Geometry check sheet. Reference: the model listing, model coordinates, mm. A direction names the side the tool comes from. Coordinates: 2 decimals unless noted, no trailing zeros. Write each loop counter-clockwise with the first axis right and the second up, starting at its lowest first coordinate (ties: lowest second). Pieces come first, ordered by that corner, then holes. Notation, with made-up numbers: M 71,66 L 80,66 A32 ccw 80,100 Z; hole C 44.5,42 d3. An arc over 180 degrees is marked long. Write item = value, one per line. Start each with the question number.
```python
from build123d import *

# Parameters (mm, degrees)
SZKIC1_R                    = 40
DODANIE_WYCI_GNI_CIE1_DEPTH = 300
DODANIE_WYCI_GNI_CIE2_DEPTH = 40
SZKIC3_R                    = 30
WYTNIJ_WYCI_GNI_CIE1_DEPTH  = 81


with BuildPart() as part:
    # Szkic1 → Dodanie-wyciągnięcie1 (new body)
    with BuildSketch(Plane.XY):
        Circle(SZKIC1_R)
    extrude(amount=DODANIE_WYCI_GNI_CIE1_DEPTH)

    # Szkic2 → Dodanie-wyciągnięcie2 (add, symmetric)
    with BuildSketch(Plane(origin=(0, 0, 0), x_dir=(0, 0, -1), z_dir=(1, 0, 0))):
        with BuildLine():
            Line((-340, -40), (-300, -40))
            Line((-300, -40), (-300, 40))
            Line((-300, 40), (-340, 40))
            ThreePointArc((-340, 40), (-380, 0), (-340, -40))
        make_face()
    extrude(amount=DODANIE_WYCI_GNI_CIE2_DEPTH, both=True)

    # Szkic3 → Wytnij-wyciągnięcie1 (cut, through all)
    with BuildSketch(Plane(origin=(40, 0, 0), x_dir=(0, 0, -1), z_dir=(1, 0, 0))):
        with Locations((-340, 0)):
            Circle(SZKIC3_R)
    extrude(amount=-WYTNIJ_WYCI_GNI_CIE1_DEPTH, mode=Mode.SUBTRACT)


solid = part.part
```
Q1. Set-up check for faces 1 (the face through (-32, 32, 300)), 2 (the face through (-8.67, -39.05, 147.9)), 3 (the face through (-30, -32, 300)), 4 (the face through (32, 30, 300)): record each of +Z, -Z, +X, -X, +Y, -Y from which the full face is reachable in a straight line by a thin tool's end or side.
Q2. Cross-section at A-A on y = -16.5. Enter the section's corners in (x, z), and give its area (3 significant figures).
Q3. Scan lines: L1, parallel to Y at x = 3, z = 340; L2, parallel to Y at x = 36, z = 358; L3, parallel to Z at x = -32.5, y = 7.5. Record each from-to range of solid material in increasing order.
Q4. Cross-section at C-C on z = 138.5. Enter the section's corners in (x, y), and give its area (3 significant figures).
Q5. Gauge pin test, flat ends, axial feed: pin 1 (3 mm diameter, centred on y = -26, z = 126, fed in from +X); pin 2 (1.5 mm diameter, centred on y = 26.5, z = 102.5, fed in from -X); pin 3 (3 mm diameter, centred on x = -31, z = 242, fed in from +Y). Record the tip position at first contact, or that the pin passes through.
Q6. Cross-section at B-B on x = -35. Enter the section's corners in (y, z), and give its area (3 significant figures).
Q7. Draft check along Z on faces 5 (the face through (0.56, 1.32, 369.97)), 6 (the face through (0.56, 0.88, 379.99)), 7 (the face through (40, -17, 314)). Enter one of: pulls with the +Z half, pulls with the -Z half, needs draft (parallel to the pull), parting line crosses it, or undercut.
Q8. Cross-section at D-D on y = 12.5. Enter the section's corners in (x, z), and give its area (3 significant figures).
Values found:
q1.face_1 = -Z, -X, +Y
q1.face_2 = -Z
q1.face_3 = -Z, -X, -Y
q1.face_4 = -Z, +X, +Y
q2.outline = M -40,300 L -36.44,300 L -36.44,0 L 36.44,0 L 36.44,300 L 40,300 L 40,314.95 L -40,314.95 Z; M -40,365.05 L 40,365.05 L 40,376.44 L -40,376.44 Z
q2.area = 24,000 mm²
q3.L1 = -40 to -30, 30 to 40
q3.L2 = -35.72 to -24, 24 to 35.72
q3.L3 = 0 to 310.95, 369.05 to 379.29
q4.outline = C 0,0 d80
q4.area = 5,030 mm²
q5.pin_1 = 31.62
q5.pin_2 = -30.61
q5.pin_3 = 27.01
q6.outline = M -40,300 L -19.36,300 L -19.36,0 L 19.36,0 L 19.36,300 L 40,300 L 40,340 A40 ccw -40,340 Z; hole C 0,340 d60
q6.area = 14,500 mm²
q7.face_5 = undercut
q7.face_6 = pulls with the +Z half
q7.face_7 = needs draft
q8.outline = M -40,300 L -38,300 L -38,0 L 38,0 L 38,300 L 40,300 L 40,312.73 L -40,312.73 Z; M -40,367.27 L 40,367.27 L 40,378 L -40,378 Z
q8.area = 24,700 mm²
